Source: CAD feature listing. Evaluate the final solid. Frame: model axes, mm. A direction names the side the tool comes from. Coordinates: 2 decimals unless noted, no trailing zeros. One line per question, with ' | ' between items. Start each with the question number.
Q1. Line query: line 1 (X direction, y = -0.45, z = 6.75) (3 decimals); line 2 (Y direction, x = 28, z = 0); line 3 (Z direction, x = 26.5, y = 39). Output: solid intervals per line, ascending.
Q2. Cut plane A-A, the plane y = -80.5. Give the number of separate pieces and of enclosed holes in the cut face, plus the area to 3 significant figures.
Q3. Draft query along Y for faces 6 (the face through (29, 9, -2)), 7 (the face through (20.105, -102.077, 4.47)), 8 (the face through (27.48, 58.66, -1.4)). Return one class per face: +Y half, -Y half, draft (parallel to the pull), parting line (faces both ways), or undercut.
Q4. Contact query for flat-ended pins moving along their axis: P1, Ø1.2, axis at x = 11, y = -93, coming from the -Z side; P2, Ø6, axis at x = 10, z = -6.5, coming from the +Y side; P3, Ø1.1, axis at x = 6.75, z = -6.75, coming from the +Y side. Output: stop coordinate, or through.
Q5. Access query for faces 1 (the face through (-23, -93, 6)), 2 (the face through (-0.322, -102.894, -4.115)), 3 (the face through (0, -37, 3)), 4 (the face through (-26, 46, 5)), 5 (the face through (-0.35, 12.73, 9.2)). Directions: +Z, -Z, +X, -X, +Y, -Y. A direction counts if a zero-diameter tool reaches every point of the face in a straight line with its end or side. Return the directions, or none.
```python
from build123d import *

# Parameters (mm, degrees)
BOSS_EXTRUDE1_DEPTH      = 4
BOSS_EXTRUDE1_DEPTH_BACK = 2
SKETCH2_W                = 50
SKETCH2_H                = 30
SKETCH3_R                = 10.75
BOSS_EXTRUDE2_DEPTH      = 4
SKETCH4_R                = 10.75
SKETCH4_R_2              = 6.25
BOSS_EXTRUDE3_DEPTH      = 1
SKETCH5_R                = 6.25
SKETCH5_R_2              = 5.01
BOSS_EXTRUDE4_DEPTH      = 1
BOSS_EXTRUDE5_START      = -1
SKETCH6_R                = 6.25
SKETCH6_R_2              = 4.875
BOSS_EXTRUDE5_DEPTH      = 1
SKETCH8_R                = 0.875
CUT_EXTRUDE1_DEPTH       = 10
SKETCH9_W                = 58
SKETCH9_H                = 24
BOSS_EXTRUDE6_DEPTH      = 4
SKETCH15_W               = 46
SKETCH15_H               = 17
BOSS_EXTRUDE7_DEPTH      = 4
BOSS_EXTRUDE8_DEPTH      = 46
SKETCH18_W               = 91.307129758
SKETCH18_H               = 96.091784827
CUT_EXTRUDE3_DEPTH       = 21
FILLET1_R                = 2
BOSS_EXTRUDE9_START      = -4
BOSS_EXTRUDE9_DEPTH      = 50
FILLET3_R                = 1
FILLET4_R                = 1


with BuildPart() as part:
    # Sketch2 → Boss-Extrude1 (new, two sides: drawn at the far end of the back side and taken through both)
    with BuildSketch(Plane(origin=(0, 0, 0), x_dir=(1, 0, 0), z_dir=(0, 1, 0)).offset(-BOSS_EXTRUDE1_DEPTH_BACK)):
        Rectangle(SKETCH2_W, SKETCH2_H)
    extrude(amount=BOSS_EXTRUDE1_DEPTH + BOSS_EXTRUDE1_DEPTH_BACK)

    # Sketch3 → Boss-Extrude2 (add)
    with BuildSketch(Plane.ZY.offset(25)):
        with BuildLine():
            Line((-15, -2), (-15, 48))
            ThreePointArc((-15, 48), (0, 63), (15, 48))
            Line((15, 48), (15, -2))
            Line((15, -2), (-15, -2))
        make_face()
        with Locations((0, 48)):
            Circle(SKETCH3_R, mode=Mode.SUBTRACT)
    boss_extrude2 = extrude(amount=BOSS_EXTRUDE2_DEPTH)

    # Mirror1: Boss-Extrude2 across plane
    add(boss_extrude2.mirror(Plane(origin=(0, 0, 0), x_dir=(0, 0, 1), z_dir=(1, 0, 0))))

    # Sketch4 → Boss-Extrude3 (add)
    with BuildSketch(Plane(origin=(-25, 0, 0), x_dir=(0, 0, -1), z_dir=(1, 0, 0))):
        with Locations((0, 48)):
            Circle(SKETCH4_R)
        with Locations((0, 48)):
            Circle(SKETCH4_R_2, mode=Mode.SUBTRACT)
    boss_extrude3 = extrude(amount=-BOSS_EXTRUDE3_DEPTH)

    # Mirror2: Boss-Extrude3 across plane
    add(boss_extrude3.mirror(Plane(origin=(0, 0, 0), x_dir=(0, 0, 1), z_dir=(1, 0, 0))))

    # Sketch5 → Boss-Extrude4 (add)
    with BuildSketch(Plane(origin=(26, 0, 0), x_dir=(0, 0, -1), z_dir=(1, 0, 0))):
        with Locations((0, 48)):
            Circle(SKETCH5_R)
        with Locations((0, 48)):
            Circle(SKETCH5_R_2, mode=Mode.SUBTRACT)
    extrude(amount=-BOSS_EXTRUDE4_DEPTH)

    # Sketch6 → Boss-Extrude5 (add)
    with BuildSketch(Plane.ZY.offset(26).offset(BOSS_EXTRUDE5_START)):
        with Locations((0, 48)):
            Circle(SKETCH6_R)
        with Locations((0, 48)):
            Circle(SKETCH6_R_2, mode=Mode.SUBTRACT)
    extrude(amount=BOSS_EXTRUDE5_DEPTH)

    # Sketch8 → Cut-Extrude1 (cut)
    with BuildSketch(Plane.XZ.offset(2)):
        with Locations(Location((-6.75, 6.75, 0), (0, 0, 270))):
            Circle(SKETCH8_R)
        with Locations(Location((6.75, 6.75, 0), (0, 0, 270))):
            Circle(SKETCH8_R)
        with Locations(Location((6.75, -6.75, 0), (0, 0, 270))):
            Circle(SKETCH8_R)
        with Locations(Location((-6.75, -6.75, 0), (0, 0, 270))):
            Circle(SKETCH8_R)
    extrude(amount=-CUT_EXTRUDE1_DEPTH, mode=Mode.SUBTRACT)



with BuildPart() as body_2:
    # Sketch9 → Boss-Extrude6 (new body)
    with BuildSketch(Plane(origin=(0, -37, 0), x_dir=(-1, 0, 0), z_dir=(0, -1, 0))):
        with Locations((0, -3)):
            Rectangle(SKETCH9_W, SKETCH9_H)
    extrude(amount=BOSS_EXTRUDE6_DEPTH)


with BuildPart() as part_1:
    add(part.part)

    add(body_2.part)  # Loft3 merges body 2
    # Sketch11 → Loft3 section 0
    with BuildSketch(Plane.XZ.offset(2)):
        with BuildLine():
            Line((-29, -15), (-21, -15))
            Line((-21, -15), (-21, -8))
            Line((-21, -8), (-29, -8))
            Line((-29, -8), (-29, -15))
        make_face()
    # Sketch10 → Loft3 section 1
    with BuildSketch(Plane.XZ.offset(41)):
        with BuildLine():
            Line((-29, -9), (-22, -9))
            Line((-22, -9), (-22, -3))
            Line((-22, -3), (-29, -3))
            Line((-29, -3), (-29, -9))
        make_face()
    loft()

    # Sketch11<6> → Loft4 section 0
    with BuildSketch(Plane.XZ.offset(2)):
        with BuildLine():
            Line((-29, 15), (-21, 15))
            Line((-21, 15), (-21, 8))
            Line((-21, 8), (-29, 8))
            Line((-29, 8), (-29, 15))
        make_face()
    # Sketch10<6> → Loft4 section 1
    with BuildSketch(Plane.XZ.offset(41)):
        with BuildLine():
            Line((-29, 15), (-22, 15))
            Line((-22, 15), (-22, 9))
            Line((-22, 9), (-29, 9))
            Line((-29, 9), (-29, 15))
        make_face()
    loft()

    # Sketch11<7> → Loft5 section 0
    with BuildSketch(Plane.XZ.offset(2)):
        with BuildLine():
            Line((29, 15), (21, 15))
            Line((21, 15), (21, 8))
            Line((21, 8), (29, 8))
            Line((29, 8), (29, 15))
        make_face()
    # Sketch10<7> → Loft5 section 1
    with BuildSketch(Plane.XZ.offset(41)):
        with BuildLine():
            Line((29, 15), (22, 15))
            Line((22, 15), (22, 9))
            Line((22, 9), (29, 9))
            Line((29, 9), (29, 15))
        make_face()
    loft()

    # Sketch11<8> → Loft6 section 0
    with BuildSketch(Plane.XZ.offset(2)):
        with BuildLine():
            Line((29, -15), (21, -15))
            Line((21, -15), (21, -8))
            Line((21, -8), (29, -8))
            Line((29, -8), (29, -15))
        make_face()
    # Sketch10<8> → Loft6 section 1
    with BuildSketch(Plane.XZ.offset(41)):
        with BuildLine():
            Line((29, -9), (22, -9))
            Line((22, -9), (22, -3))
            Line((22, -3), (29, -3))
            Line((29, -3), (29, -9))
        make_face()
    loft()

    # Sketch14 → Loft7 section 0
    with BuildSketch(Plane.XZ.offset(41)):
        with BuildLine():
            Line((-29, -9), (-21, -9))
            Line((-21, -9), (-21, -2))
            Line((-21, -2), (-29, -2))
            Line((-29, -2), (-29, -9))
        make_face()
    # Sketch13 → Loft7 section 1
    with BuildSketch(Plane(origin=(0, -91, 0), x_dir=(-1, 0, 0), z_dir=(0, -1, 0))):
        with BuildLine():
            Line((23, 2), (15, 2))
            Line((15, 2), (15, -3))
            Line((15, -3), (23, -3))
            Line((23, -3), (23, 2))
        make_face()
    loft()

    # Loft8: read off the stored shape, not the designer's step
    # Loft8: loft between two sections, ruled curve by curve
    loft8_from = [
        Edge.make_line((21, -41, -2), (29, -41, -2)),
        Edge.make_line((29, -41, -2), (29, -41, -9)),
        Edge.make_line((21, -41, -9), (21, -41, -2)),
        Edge.make_line((21, -41, -9), (29, -41, -9)),
    ]
    loft8_to = [
        Edge.make_line((15, -91, 3), (23, -91, 3)),
        Edge.make_line((23, -91, 3), (23, -91, -2)),
        Edge.make_line((15, -91, -2), (15, -91, 3)),
        Edge.make_line((15, -91, -2), (23, -91, -2)),
    ]
    loft8 = Solid(Shell([*[Face.make_surface_from_curves(loft8_from[k], loft8_to[k]) for k in range(4)], Face(Wire(loft8_from)), Face(Wire(loft8_to))]))
    add(loft8)

    # Loft9: read off the stored shape, not the designer's step
    # Loft9: loft between two sections, ruled curve by curve
    loft9_from = [
        Edge.make_line((29, -41, 15), (29, -41, 8)),
        Edge.make_line((21, -41, 8), (21, -41, 15)),
        Edge.make_line((29, -41, 8), (21, -41, 8)),
        Edge.make_line((21, -41, 15), (29, -41, 15)),
    ]
    loft9_to = [
        Edge.make_line((23, -91, 15), (23, -91, 10)),
        Edge.make_line((15, -91, 10), (15, -91, 15)),
        Edge.make_line((23, -91, 10), (15, -91, 10)),
        Edge.make_line((15, -91, 15), (23, -91, 15)),
    ]
    loft9 = Solid(Shell([*[Face.make_surface_from_curves(loft9_from[k], loft9_to[k]) for k in range(4)], Face(Wire(loft9_from)), Face(Wire(loft9_to))]))
    add(loft9)

    # Loft10: read off the stored shape, not the designer's step
    # Loft10: loft between two sections, ruled curve by curve
    loft10_from = [
        Edge.make_line((-21, -41, 15), (-21, -41, 8)),
        Edge.make_line((-29, -41, 8), (-29, -41, 15)),
        Edge.make_line((-21, -41, 8), (-29, -41, 8)),
        Edge.make_line((-29, -41, 15), (-21, -41, 15)),
    ]
    loft10_to = [
        Edge.make_line((-15, -91, 15), (-15, -91, 10)),
        Edge.make_line((-23, -91, 10), (-23, -91, 15)),
        Edge.make_line((-15, -91, 10), (-23, -91, 10)),
        Edge.make_line((-23, -91, 15), (-15, -91, 15)),
    ]
    loft10 = Solid(Shell([*[Face.make_surface_from_curves(loft10_from[k], loft10_to[k]) for k in range(4)], Face(Wire(loft10_from)), Face(Wire(loft10_to))]))
    add(loft10)

    # Sketch15 → Boss-Extrude7 (add)
    with BuildSketch(Plane.XZ.offset(91)):
        with Locations((0, 6.5)):
            Rectangle(SKETCH15_W, SKETCH15_H)
    extrude(amount=BOSS_EXTRUDE7_DEPTH)

    # Sketch16 → Boss-Extrude8 (add)
    with BuildSketch(Plane.ZY.offset(23)):
        Polygon((15, -95), (-2, -95), (-8.222431864, -118.222431864), align=None)
        Polygon((-2.426876907, -108.184236219), (0.301980964, -98), (7.757359313, -98), align=None, mode=Mode.SUBTRACT)
    extrude(amount=-BOSS_EXTRUDE8_DEPTH)

    # Sketch18 → Cut-Extrude3 (cut)
    with BuildSketch(Plane(origin=(-52.994526892, -21.679383469, 0), x_dir=(0, 0, -1), z_dir=(0.9255481540620362, 0.37862991761396436, 0))):
        with Locations((11.5562698, -126.796989603)):
            Rectangle(SKETCH18_W, SKETCH18_H)
    cut_extrude3 = extrude(amount=-CUT_EXTRUDE3_DEPTH, mode=Mode.SUBTRACT)

    # Mirror3: Cut-Extrude3 across plane
    add(cut_extrude3.mirror(Plane.ZY), mode=Mode.SUBTRACT)

    # Fillet1
    fillet1_edges = [part_1.edges().sort_by_distance(p)[0] for p in [
        (0, -118.222431864, -8.222431864),
    ]]
    fillet(fillet1_edges, radius=FILLET1_R)

    # Sketch22 → Boss-Extrude9 (add)
    with BuildSketch(Plane.ZY.offset(29).offset(BOSS_EXTRUDE9_START)):
        Polygon((14.968137022, 3.610533067), (9.468137022, 3.610533067), (4.968137022, 3.610533067), (15, 25.228846085), (14.968137022, 3.960925502), align=None)
    extrude(amount=-BOSS_EXTRUDE9_DEPTH)

    # Fillet3
    fillet3_edges = [part_1.edges().sort_by_distance(p)[0] for p in [
        (0, 4, 5.148867077),
    ]]
    fillet(fillet3_edges, radius=FILLET3_R)

    # Fillet4
    fillet4_edges = [part_1.edges().sort_by_distance(p)[0] for p in [
        (0, 25.228846085, 15),
    ]]
    fillet(fillet4_edges, radius=FILLET4_R)


solid = part_1.part
```
Reply:
1) line 1: x = -29 to -7.625, -5.875 to 5.875, 7.625 to 29 | line 2: y = -41 to -37, -2 to 37.25, 58.75 to 63 | line 3: z = -15 to -5.88, 5.88 to 15
2) separate pieces: 4 | enclosed holes: 0 | area: 173 mm^2
3) face 6: draft | face 7: -Y half | face 8: undercut
4) P1: stops at z = -2 | P2: stops at y = 4 | P3: stops at y = -37
5) face 1: +Z, -Z, -X, -Y | face 2: -Z, +X, -X | face 3: none | face 4: -X | face 5: -Z, +Y
